Design review of the part shown in the three views and the two pictorial views. Dimensions are in mm from the part's minimum x, y and z. A direction names the side the tool comes from. Coordinates: 2 decimals unless noted, no trailing zeros. Write each loop counter-clockwise with the first axis right and the second up, starting at its lowest first coordinate (ties: lowest second). Pieces come first, ordered by that corner, then holes. Notation, with made-up numbers: M 4.25,74.5 L 53.25,74.5 A11 cw 53.25,85.5 Z; hole C 62.25,7.25 d6. An arc over 180 degrees is marked long. One line per question, with ' | ' between items.
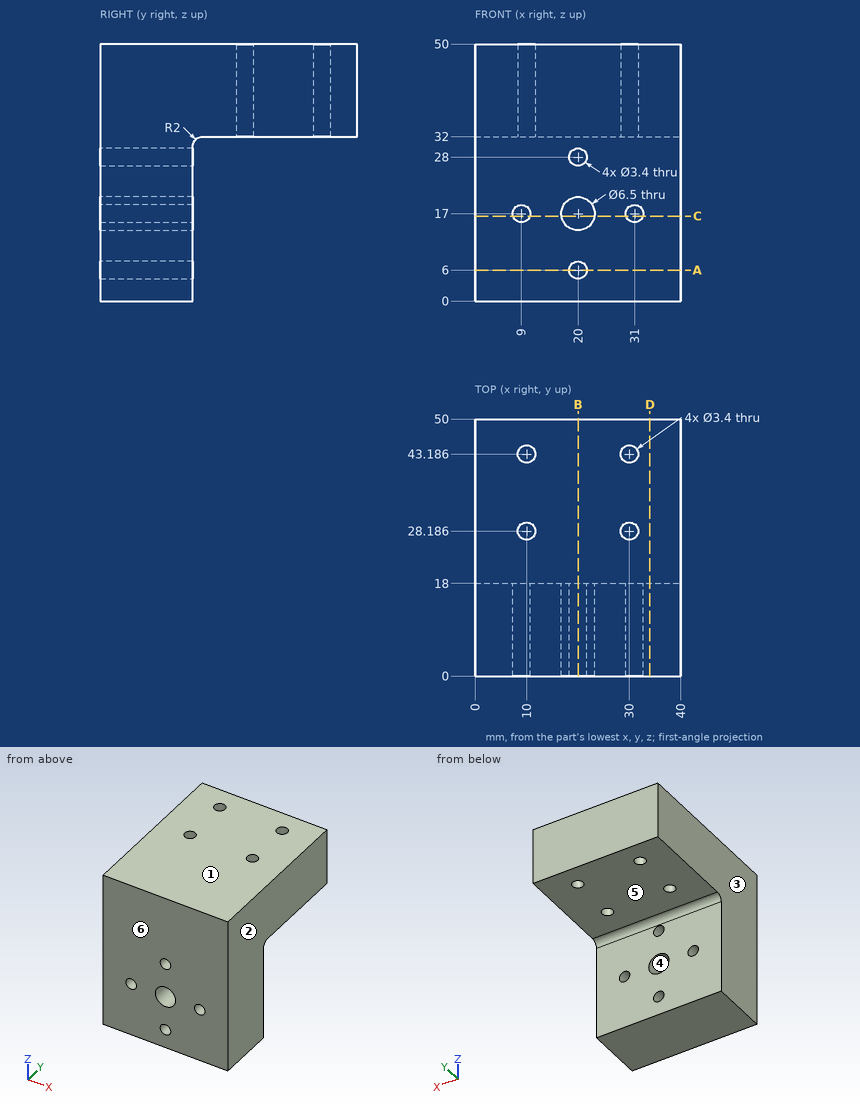
1. Machinability: for the marked faces 5 and 6, which of the approach directions +Z, -Z, +X, -X, +Y, -Y give a long, thin tool a straight path to every point of the face, cutting with its end or side? Answer none if there is none.
Computed values:
face 5: -Z, +X, -X, +Y | face 6: +Z, -Z, +X, -X, -Y
2. Take a section at B-B on x = 20. State the section outline as (y, z) points, plus the area to 3 significant figures.
Computed values:
outline: M 0,0 L 18,0 L 18,4.3 L 0,4.3 Z; M 0,7.7 L 18,7.7 L 18,13.75 L 0,13.75 Z; M 0,20.25 L 18,20.25 L 18,26.3 L 0,26.3 Z; M 0,29.7 L 18,29.7 L 18,30 A2 cw 20,32 L 50,32 L 50,50 L 0,50 Z | area: 1,240 mm2
3. Take a section at A-A on z = 6. State the section outline as (x, y) points.
Computed values:
outline: M 0,0 L 18.3,0 L 18.3,18 L 0,18 Z; M 21.7,0 L 40,0 L 40,18 L 21.7,18 Z
4. For line 1 along X through (y, z) = (11, 17); line 2 along Y through (x, z) = (11.5, 37) (1 decimal); line 3 along Y through (x, z) = (2, 13.5), list the stretches that pass through material, from the lowest coordinate up.
Computed values:
line 1: x = 0 to 7.3, 10.7 to 16.75, 23.25 to 29.3, 32.7 to 40 | line 2: y = 0 to 27.4, 29 to 42.4, 44 to 50 | line 3: y = 0 to 18
5. Take a section at D-D on x = 34. State the section outline as (y, z) points.
Computed values:
outline: M 0,0 L 18,0 L 18,30 A2 cw 20,32 L 50,32 L 50,50 L 0,50 Z
6. Clearance check with flat-ended pins moving along their axes: P1, Ø2, axis at x = 24.5, y = 34.5, coming from the -Z side; P2, Ø24, axis at x = 21.5, z = 12.5, coming from the +Y side; P3, Ø5, axis at x = 7, z = 28, coming from the +Y side. State where each tip first meets the part, or that it passes through.
Computed values:
P1: stops at z = 32 | P2: stops at y = 18 | P3: stops at y = 18.06
7. Draft analysis for pull direction X (two halves, no side actions). For the marked faces 1, 2, 3 and 4, state which applies: pulls with the +X half, pulls with the -X half, needs draft (parallel to the pull), parting line crosses it, or undercut.
Computed values:
face 1: needs draft | face 2: pulls with the +X half | face 3: pulls with the -X half | face 4: undercut
8. Take a section at C-C on z = 16.5. State the section outline as (x, y) points (1 decimal), plus the area to 3 significant figures.
Computed values:
outline: M 0,0 L 7.4,0 L 7.4,18 L 0,18 Z; M 10.6,0 L 16.8,0 L 16.8,18 L 10.6,18 Z; M 23.2,0 L 29.4,0 L 29.4,18 L 23.2,18 Z; M 32.6,0 L 40,0 L 40,18 L 32.6,18 Z | area: 487 mm2
